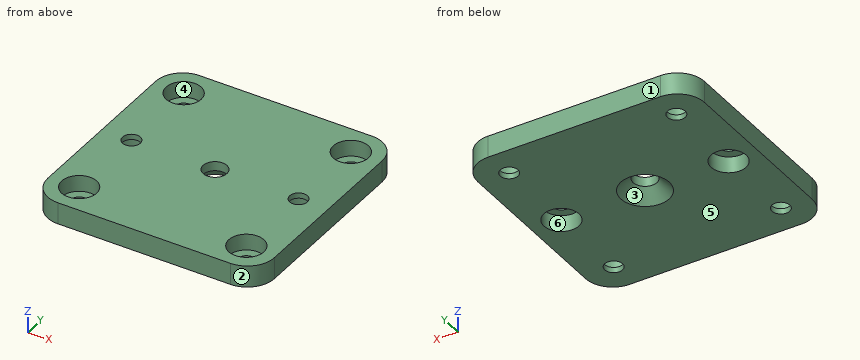
```python
from build123d import *

# Parameters (mm, degrees)
F0_W           = 42
F0_H           = 42
F1_DEPTH       = 4
F3_R           = 5
F4_D           = 3.3
F4_CBORE_D     = 6.5
F4_CBORE_DEPTH = 3
F6_D           = 4.4
F6_CSINK_D     = 8.96
F6_CSINK_ANGLE = 90
F8_D           = 3.3
F8_CBORE_D     = 6.5
F8_CBORE_DEPTH = 3


with BuildPart() as f1:
    # F0 (on Top) → F1 (new body)
    with BuildSketch(Plane.XY):
        Rectangle(F0_W, F0_H)
    extrude(amount=F1_DEPTH)

    # F3
    f3_edges = [f1.edges().sort_by_distance(p)[0] for p in [
        (-21, 21, 2),
        (-21, -21, 2),
        (21, -21, 2),
        (21, 21, 2),
    ]]
    fillet(f3_edges, radius=F3_R)

    # F4 (through all)
    with Locations(Plane.XY.offset(4)):
        with Locations((-15.5, 15.5), (15.5, 15.5), (15.5, -15.5), (-15.5, -15.5)):
            CounterBoreHole(F4_D / 2, F4_CBORE_D / 2, F4_CBORE_DEPTH)

    # F6 (through all)
    with Locations(Plane(origin=(0, 0, 0), x_dir=(1, 0, 0), z_dir=(0, 0, -1))):
        with Locations((0, 0)):
            CounterSinkHole(F6_D / 2, F6_CSINK_D / 2, counter_sink_angle=F6_CSINK_ANGLE)

    # F8 (through all)
    with Locations(Plane(origin=(0, 0, 0), x_dir=(1, 0, 0), z_dir=(0, 0, -1))):
        with Locations((-15.5, 0), (15.5, 0)):
            CounterBoreHole(F8_D / 2, F8_CBORE_D / 2, F8_CBORE_DEPTH)


solid = f1.part
```
For this review, take the finished solid that the model builds, in its own axes (mm). Face numbers are marked on the shaded views. A direction names the side the tool comes from. Round coordinates to 2 decimals unless told otherwise and drop trailing zeros. Order: outer loops, then holes, each group sorted by start corner. A loop starts at its lowest first (then second) coordinate and runs counter-clockwise, first axis right, second up.
Q1. We need section B-B, the plane x = -15.5. Give the boundary of the cut face in (y, z), plus the area to 3 significant figures.
Findings below:
outline: (-21, 0) - (-17.15, 0) - (-17.15, 1) - (-18.75, 1) - (-18.75, 4) - (-21, 4) - close; (-13.85, 0) - (-3.25, 0) - (-3.25, 3) - (-1.65, 3) - (-1.65, 4) - (-12.25, 4) - (-12.25, 1) - (-13.85, 1) - close; (1.65, 3) - (3.25, 3) - (3.25, 0) - (13.85, 0) - (13.85, 1) - (12.25, 1) - (12.25, 4) - (1.65, 4) - close; (17.15, 0) - (21, 0) - (21, 4) - (18.75, 4) - (18.75, 1) - (17.15, 1) - close
area: 99.6 mm2
Q2. Wall thickness on line 1 (Y direction, x = -15.5, z = 3.2); line 2 (Y direction, x = -17, z = 1.25); line 3 (X direction, y = -18.5, z = 3.1): over which ranges is each line inside the solid? List them lowest first.
Findings below:
line 1: y = -21 to -18.75, -12.25 to -1.65, 1.65 to 12.25, 18.75 to 21
line 2: y = -20.9 to -18.38, -12.62 to -2.88, 2.88 to 12.62, 18.38 to 20.9
line 3: x = -20.33 to -16.75, -14.25 to 14.25, 16.75 to 20.33
Q3. We need section D-D, the plane y = 15.5. Give the boundary of the cut face in (x, z), plus the area to 3 significant figures.
Findings below:
outline: (-21, 0) - (-17.15, 0) - (-17.15, 1) - (-18.75, 1) - (-18.75, 4) - (-21, 4) - close; (-13.85, 0) - (13.85, 0) - (13.85, 1) - (12.25, 1) - (12.25, 4) - (-12.25, 4) - (-12.25, 1) - (-13.85, 1) - close; (17.15, 0) - (21, 0) - (21, 4) - (18.75, 4) - (18.75, 1) - (17.15, 1) - close
area: 122 mm2
Q4. Machinability: for the marked faces 4, 5 and 6, which of the approach directions +Z, -Z, +X, -X, +Y, -Y give a long, thin tool a straight path to every point of the face, cutting with its end or side? Answer none if there is none.
Findings below:
face 4: +Z
face 5: -Z, +X, -X, +Y, -Y
face 6: -Z
Q5. We need section A-A, the plane x = 0. Give the boundary of the cut face in (y, z).
Findings below:
outline: (-21, 0) - (-4.48, 0) - (-2.2, 2.28) - (-2.2, 4) - (-21, 4) - close; (2.2, 2.28) - (4.48, 0) - (21, 0) - (21, 4) - (2.2, 4) - close
Q6. Insertion check: P1, Ø3, axis at x = -15.5, y = 17, coming from the +Z side. The pin has a flat end and moves straight along its axis. Give the tip position at first contact, or say it passes through.
Findings below:
P1: stops at z = 1
Q7. We need section C-C, the plane y = -14.5. Give the boundary of the cut face in (x, z).
Findings below:
outline: (-21, 0) - (-16.81, 0) - (-16.81, 1) - (-18.59, 1) - (-18.59, 4) - (-21, 4) - close; (-14.19, 0) - (14.19, 0) - (14.19, 1) - (12.41, 1) - (12.41, 4) - (-12.41, 4) - (-12.41, 1) - (-14.19, 1) - close; (16.81, 0) - (21, 0) - (21, 4) - (18.59, 4) - (18.59, 1) - (16.81, 1) - close
Q8. Mouldability with a two-part tool opening along Y and no side actions: class the marked faces 1, 2 and 3 as pulls with the +Y half, pulls with the -Y half, needs draft (parallel to the pull), parting line crosses it, or undercut.
Findings below:
face 1: pulls with the +Y half
face 2: pulls with the -Y half
face 3: undercut
